Build history of the part. All positions in model axes, mm. Round coordinates to 2 decimals unless told otherwise and drop trailing zeros. Write each loop counter-clockwise with the first axis right and the second up, starting at its lowest first coordinate (ties: lowest second). Pieces come first, ordered by that corner, then holes. Notation, with made-up numbers: (86.25, 44) - (111.25, 44) arc R5 cw to (111.25, 53) - close; hole circle Ø11 at (74, -31). An arc over 180 degrees is marked (long way). Write each question's results on one line, items separated by ' | '.
Autodesk Inventor part; units mm, degrees
ref_plane "YZ Plane" through (0, 0, 0) normal (1, 0, 0) x (0, 1, 0)
ref_plane "XZ Plane" through (0, 0, 0) normal (0, 1, 0) x (-1, 0, 0)
ref_plane "XY Plane" through (0, 0, 0) normal (0, 0, 1) x (1, 0, 0)
sketch "Sketch1" plane through (0, 0, 0) normal (0, 0, 1) x (1, 0, 0)
  line L0 (-10, -10) -> (10, -10)
  line L1 (10, -10) -> (10, 10)
  line L2 (10, 10) -> (-10, 10)
  line L3 (-10, 10) -> (-10, -10)
  line L4 (-10, -10) -> (10, 10) construction
  line L5 (10, -10) -> (-10, 10) construction
  point P0 (0, 0)
  dimension "d0" = 20
  dimension "d1" = 20
extrude "Extrusion1" add sketch "Sketch1" along normal blind 2
chamfer "Chamfer1" distance 1 angle 45 1 edges at (0, 10, 2)
chamfer "Chamfer2" distance 1 angle 45 3 edges at (10, -0.5, 2) (-10, -0.5, 2) (0, -10, 2)
properties part number "Bit Nhom 3060"
(1) Slice it at B-B, the plane z = 1.35. Write the cut outline in (x, y).
Worked answers:
outline: (-9.65, -9.65) - (9.65, -9.65) - (9.65, 9.65) - (-9.65, 9.65) - close
(2) Flat gauge pin, fed straight in: pin 1 Ø1 at (x, y) = (-6.5, -7.5) entering from -Z. Where does the tip first touch, or does it go through?
Worked answers:
pin 1: stops at z = 0
(3) Slice it at A-A, the plane x = 2. Write the cut outline in (y, z).
Worked answers:
outline: (-10, 0) - (10, 0) - (10, 1) - (9, 2) - (-9, 2) - (-10, 1) - close
(4) Drill centre lines: probe 1 along Y at (x, z) = (5, 1.25); probe 2 along X at (y, z) = (-2, 1.45); probe 3 along X at (y, z) = (0.75, 1.4). Where is each one in solid material? Low to high. Write a range as [from, to].
Worked answers:
probe 1: y = [-9.75, 9.75] | probe 2: x = [-9.55, 9.55] | probe 3: x = [-9.6, 9.6]
